Could you check a few things on this model? Use its own coordinates, in mm. A direction names the side the tool comes from. Coordinates: 2 decimals unless noted, no trailing zeros. Loops run counter-clockwise (first coordinate to the right, second up) from the corner with the lowest first, then second, coordinate; pieces in that order, holes last. Notation, with made-up numbers: (77, 0) -> (84, 0) arc R24 ccw to (84, 16) -> close; hole circle Ø2 at (70, 16). An arc over 180 degrees is marked (long way). One line per question, with ' | ' between items.
Autodesk Inventor part; units mm, degrees
ref_plane "pin_XY" through (0, 0, 0) normal (1, 0, 0) x (0, 0, -1)
ref_plane "pin_YZ" through (0, 0, 0) normal (0, 0, -1) x (0, 1, 0)
ref_plane "pin_ZX" through (0, 0, 0) normal (0, 1, 0) x (1, 0, 0)
sketch "Sketch_1" plane through (0, 0, 0) normal (0, 0, 1) x (1, 0, 0)
  line L0 (6.2865, 0) -> (-6.2865, 0)
  line L1 (-6.2865, 0) -> (-6.2865, 1.2065)
  line L2 (-6.2865, 1.2065) -> (-5.9055, 1.5875)
  line L3 (-5.9055, 1.5875) -> (-4.9403, 1.5875)
  line L4 (-4.9403, 1.5875) -> (-4.9403, 1.2827)
  arc A0 (-4.9403, 1.2827) -> (-4.8768, 1.2192) centre (-4.8768, 1.2827) ccw
  line L5 (-4.8768, 1.2192) -> (-4.5212, 1.2192)
  arc A1 (-4.5212, 1.2192) -> (-4.4577, 1.2827) centre (-4.5212, 1.2827) ccw
  line L6 (-4.4577, 1.2827) -> (-4.4577, 1.5875)
  line L7 (-4.4577, 1.5875) -> (4.4577, 1.5875)
  line L8 (4.4577, 1.5875) -> (4.4577, 1.2827)
  arc A2 (4.4577, 1.2827) -> (4.5212, 1.2192) centre (4.5212, 1.2827) ccw
  line L9 (4.5212, 1.2192) -> (4.8768, 1.2192)
  arc A3 (4.8768, 1.2192) -> (4.9403, 1.2827) centre (4.8768, 1.2827) ccw
  line L10 (4.9403, 1.2827) -> (4.9403, 1.5875)
  line L11 (4.9403, 1.5875) -> (5.9055, 1.5875)
  line L12 (5.9055, 1.5875) -> (6.2865, 1.2065)
  line L13 (6.2865, 1.2065) -> (6.2865, 0)
  line L14 (6.2865, 0) -> (-6.2865, 0)
revolve "Revolution1" add sketch "Sketch_1" angle 360 about axis through (6.2865, 0, 0) along (1, 0, 0)
ref_plane "pin_XY" through (0, 0, 0) normal (1, 0, 0) x (0, 0, -1)
ref_plane "pin_YZ" through (0, 0, 0) normal (0, 0, -1) x (0, 1, 0)
ref_plane "pin_ZX" through (0, 0, 0) normal (0, 1, 0) x (1, 0, 0)
ref_plane "rr1_XY" through (4.699, 0, 0) normal (1, 0, 0) x (0, 0, -1)
ref_plane "rr1_YZ" through (4.699, 0, 0) normal (0, 0, -1) x (0, 1, 0)
ref_plane "rr1_ZX" through (4.699, 0, 0) normal (0, 1, 0) x (1, 0, 0)
ref_plane "rr2_XY" through (-4.699, 0, 0) normal (1, 0, 0) x (0, 0, -1)
ref_plane "rr2_YZ" through (-4.699, 0, 0) normal (0, 0, -1) x (0, 1, 0)
ref_plane "rr2_ZX" through (-4.699, 0, 0) normal (0, 1, 0) x (1, 0, 0)
ref_plane "w21_XY" through (6.2865, 0, 0) normal (0, 1, 0) x (1, 0, 0)
ref_plane "w21_YZ" through (6.2865, 0, 0) normal (1, 0, 0) x (0, 0, -1)
ref_plane "w21_ZX" through (6.2865, 0, 0) normal (0, 0, -1) x (0, 1, 0)
ref_plane "w22_XY" through (-6.2865, 0, 0) normal (0, 1, 0) x (1, 0, 0)
ref_plane "w22_YZ" through (-6.2865, 0, 0) normal (1, 0, 0) x (0, 0, -1)
ref_plane "w22_ZX" through (-6.2865, 0, 0) normal (0, 0, -1) x (0, 1, 0)
ref_plane "p1_XY" through (0, 0, 1.5875) normal (1, 0, 0) x (0, 0, -1)
ref_plane "p1_YZ" through (0, 0, 1.5875) normal (0, 0, -1) x (0, 1, 0)
ref_plane "p1_ZX" through (0, 0, 1.5875) normal (0, 1, 0) x (1, 0, 0)
ref_plane "p2_XY" through (0, 0, -1.5875) normal (1, 0, 0) x (0, 0, -1)
ref_plane "p2_YZ" through (0, 0, -1.5875) normal (0, 0, -1) x (0, 1, 0)
ref_plane "p2_ZX" through (0, 0, -1.5875) normal (0, 1, 0) x (1, 0, 0)
properties part number "D-25368"
1) On a 3-axis mill with a long thin cutter (end or side, diameter ignored), from which of +Z, -Z, +X, -X, +Y, -Y can I reach the whole of each face in a straight line? I mean faces 4 (the face through (-4.7, 1.16, 0.37)), 5 (the face through (-5.42, -0.34, -1.55)). Say none if no direction works.
Data:
face 4: none | face 5: +X, -X
2) I need wall thicknesses on line 1 along X through (y, z) = (0.4, -1.2); line 2 along X through (y, z) = (-1.1, 0.95); line 3 along Y through (x, z) = (-1.5, -0.15). Which ranges of each line are inside material? Lowest first, please. Write a range as from..to.
Data:
line 1: -6.23..-4.94, -4.46..4.46, 4.94..6.23 | line 2: -6.04..-4.94, -4.46..4.46, 4.94..6.04 | line 3: -1.58..1.58
3) We'd pull the mould along X, two halves only. Please class faces 1 (the face through (6.286, 0, 0)), 2 (the face through (5.43, -0.34, -1.55)), 3 (the face through (4.7, 1.16, 0.37)): pulls with the +X half, pulls with the -X half, needs draft (parallel to the pull), parting line crosses it, or undercut.
Data:
face 1: pulls with the +X half | face 2: needs draft | face 3: undercut
4) If we section it at C-C on x = -3.75: Please give me the cut outline in (y, z) (1 decimal), and give its area (3 significant figures).
Data:
outline: circle Ø3.2 at (0, 0) | area: 7.92 mm²
